Autodesk Inventor part; units mm, degrees
ref_plane "screw_XY" through (0, 0, 0) normal (0, 1, 0) x (1, 0, 0)
ref_plane "screw_YZ" through (0, 0, 0) normal (1, 0, 0) x (0, 0, -1)
ref_plane "screw_ZX" through (0, 0, 0) normal (0, 0, -1) x (0, 1, 0)
sketch "Sketch_3" plane through (0, 0, 0) normal (0, 0, 1) x (1, 0, 0)
  line L0 (0, -1.9608) -> (0, 0.1172)
  line L1 (0, 0.1172) -> (2.413, 0.1172)
  line L2 (2.413, 0.1172) -> (4.8895, -1.9608)
  line L3 (4.8895, -1.9608) -> (0, -1.9608)
  line L4 (0, -1.9608) -> (0, 0.1172)
revolve "Revolution1" add sketch "Sketch_3" angle 360 about axis through (0, -1.9608, 0) along (0, -1, 0)
sketch "Sketch_4" plane through (0, -1.9608, 0) normal (0, -1, 0) x (1, 0, 0)
  line L0 (-2.5883, 0.5283) -> (-2.5883, -0.5283)
  line L1 (-2.5883, -0.5283) -> (-0.7823, -0.5283)
  arc A0 (-0.5283, -0.7823) -> (-0.7823, -0.5283) centre (-0.7823, -0.7823) ccw
  line L2 (-0.5283, -0.7823) -> (-0.5283, -2.5883)
  line L3 (-0.5283, -2.5883) -> (0.5283, -2.5883)
  line L4 (0.5283, -2.5883) -> (0.5283, -0.7823)
  arc A1 (0.7823, -0.5283) -> (0.5283, -0.7823) centre (0.7823, -0.7823) ccw
  line L5 (0.7823, -0.5283) -> (2.5883, -0.5283)
  line L6 (2.5883, -0.5283) -> (2.5883, 0.5283)
  line L7 (2.5883, 0.5283) -> (0.7823, 0.5283)
  arc A2 (0.5283, 0.7823) -> (0.7823, 0.5283) centre (0.7823, 0.7823) ccw
  line L8 (0.5283, 0.7823) -> (0.5283, 2.5883)
  line L9 (0.5283, 2.5883) -> (-0.5283, 2.5883)
  line L10 (-0.5283, 2.5883) -> (-0.5283, 0.7823)
  arc A3 (-0.7823, 0.5283) -> (-0.5283, 0.7823) centre (-0.7823, 0.7823) ccw
  line L11 (-0.7823, 0.5283) -> (-2.5883, 0.5283)
extrude "Extrusion1" cut sketch "Sketch_4" against normal blind 0.9195
ref_plane "screw_XY" through (0, 0, 0) normal (0, 1, 0) x (1, 0, 0)
ref_plane "screw_YZ" through (0, 0, 0) normal (1, 0, 0) x (0, 0, -1)
ref_plane "screw_ZX" through (0, 0, 0) normal (0, 0, -1) x (0, 1, 0)
properties part number "3628_"
Geometry: final body of the model. Coordinates: model frame, mm. A direction names the side the tool comes from. Coordinates: 2 decimals unless noted, no trailing zeros. Order: outer loops, then holes, each group sorted by start corner. A loop starts at its lowest first (then second) coordinate and runs counter-clockwise, first axis right, second up. Notation, with made-up numbers: (66, 72) -> (76, 72) arc R16 ccw to (76, 79) -> close; hole circle Ø1 at (26.25, -24). An arc over 180 degrees is marked (long way). Write each question's results on one line, items separated by ' | '. Start each with the question number.
1) Cut plane C-C, the plane y = -1.2. Output: boundary loops of the cut face in (x, z), and give its area (3 significant figures).
2) Cut plane B-B, the plane z = 0. Output: boundary loops of the cut face in (x, y), and give its area (3 significant figures).
3) Mould query, pull axis X, two halves, no side actions, for faces 3 (the conical face through (-0.557, -0.013, -2.507)), 4 (the flat face through (-0.528, -1.5, 1.7)), 5 (the flat face through (1, -1.961, -1)), 6 (the flat face through (0, -1.5, 2.588)). Classes: released by +X, released by -X, zero draft, split by the parting line, or undercut.
4) Material intervals for line 1 along X through (y, z) = (-1.7, -0.75); line 2 along X through (y, z) = (-1.55, -0.75); line 3 along Z through (x, y) = (-1.5, -1.6), sorted ascending.
5) Set-up query: faces 1 (the flat face through (0.528, -1.5, -1.7)), 2 (the flat face through (0, 0.117, 0)). Return all of +Z, -Z, +X, -X, +Y, -Y with unobstructed straight access to the full face (end or side cutting, diameter ignored); none if empty.
6) Cut plane D-D, the plane y = -0.1. Output: boundary loops of the cut face in (x, z), and give its area (3 significant figures).
7) Cut plane A-A, the plane x = 0. Output: boundary loops of the cut face in (y, z), and give its area (3 significant figures).
8) First-contact query: pin 1 (0.5 mm diameter, centred on y = -1.5, z = -1.5, fed in from -X); pin 2 (0.5 mm diameter, centred on y = -1.5, z = 0, fed in from +X); pin 3 (0.5 mm diameter, centred on y = -1.5, z = -1.5, fed in from +X); pin 4 (1.5 mm diameter, centred on x = -0.5, z = 1, fed in from -Y). Flat tips, straight axial feed; report the tip coordinate or a pass-through.
Checks:
1) outline: circle Ø7.97 at (0, 0); hole (-2.59, -0.53) -> (-0.78, -0.53) arc R0.25 cw to (-0.53, -0.78) -> (-0.53, -2.59) -> (0.53, -2.59) -> (0.53, -0.78) arc R0.25 cw to (0.78, -0.53) -> (2.59, -0.53) -> (2.59, 0.53) -> (0.78, 0.53) arc R0.25 cw to (0.53, 0.78) -> (0.53, 2.59) -> (-0.53, 2.59) -> (-0.53, 0.78) arc R0.25 cw to (-0.78, 0.53) -> (-2.59, 0.53) -> close | area: 40.0 mm^2
2) outline: (-4.89, -1.96) -> (-2.59, -1.96) -> (-2.59, -1.04) -> (2.59, -1.04) -> (2.59, -1.96) -> (4.89, -1.96) -> (2.41, 0.12) -> (-2.41, 0.12) -> close | area: 10.4 mm^2
3) face 3: split by the parting line | face 4: undercut | face 5: zero draft | face 6: undercut
4) line 1: -4.52 to -0.53, 0.53 to 4.52 | line 2: -4.34 to -0.53, 0.53 to 4.34 | line 3: -4.2 to -0.53, 0.53 to 4.2
5) face 1: -Y | face 2: +Z, -Z, +X, -X, +Y
6) outline: circle Ø5.34 at (0, 0) | area: 22.4 mm^2
7) outline: (-1.96, -4.89) -> (0.12, -2.41) -> (0.12, 2.41) -> (-1.96, 4.89) -> (-1.96, 2.59) -> (-1.04, 2.59) -> (-1.04, -2.59) -> (-1.96, -2.59) -> close | area: 10.4 mm^2
8) pin 1: x = -4.4 | pin 2: x = 4.64 | pin 3: x = 4.4 | pin 4: y = -1.96
